```python
from build123d import *

# Parameters (mm, degrees)
F1_DEPTH = 50
F3_R     = 5
F4_DEPTH = 5
F5_DEPTH = 3


with BuildPart() as f1:
    # F0 (on Front) → F1 (new body)
    with BuildSketch(Plane.XZ):
        Polygon((86.1805300464, 183.2075325962), (81.2134853671, 183.7806531362), (60.0080253898, 0), (64.9750700692, -0.5731205399), align=None)
    extrude(amount=-F1_DEPTH)

    # F3 (on offset) → F4 (join)
    with BuildSketch(Plane.XZ.offset(-3)):
        with BuildLine():
            Line((45.1068913518, 1.7193616198), (60.0080253898, 0))
            Line((60.0080253898, 0), (63.4467486294, 29.8022680761))
            Line((63.4467486294, 29.8022680761), (48.5456145913, 31.5216296959))
            ThreePointArc((48.5456145913, 31.5216296959), (37.5053321271, 28.3729607019), (31.925118881, 18.3398568227))
            ThreePointArc((31.925118881, 18.3398568227), (35.0737879275, 7.2995748134), (45.1068913518, 1.7193616198))
        make_face()
        with Locations((46.8262529715, 16.6204956578)):
            Circle(F3_R, mode=Mode.SUBTRACT)
    extrude(amount=-F4_DEPTH)

    # F3 (on offset) → F5 (join)
    with BuildSketch(Plane.XZ.offset(-3)):
        with BuildLine():
            Line((45.1068913518, 1.7193616198), (60.0080253898, 0))
            Line((60.0080253898, 0), (63.4467486294, 29.8022680761))
            Line((63.4467486294, 29.8022680761), (48.5456145913, 31.5216296959))
            ThreePointArc((48.5456145913, 31.5216296959), (37.5053321271, 28.3729607019), (31.925118881, 18.3398568227))
            ThreePointArc((31.925118881, 18.3398568227), (35.0737879275, 7.2995748134), (45.1068913518, 1.7193616198))
        make_face()
        with Locations((46.8262529715, 16.6204956578)):
            Circle(F3_R, mode=Mode.SUBTRACT)
        with BuildLine():
            Line((48.5456145913, 31.5216296959), (63.4467486294, 29.8022680761))
            Line((63.4467486294, 29.8022680761), (81.2134853671, 183.7806531362))
            Line((81.2134853671, 183.7806531362), (51.411217291, 187.2193763757))
            Line((51.411217291, 187.2193763757), (31.925118881, 18.3398568227))
            ThreePointArc((31.925118881, 18.3398568227), (37.5053321271, 28.3729607019), (48.5456145913, 31.5216296959))
        make_face()
    extrude(amount=F5_DEPTH)


solid = f1.part
```
Geometry check sheet. Reference: the model listing, model coordinates, mm. Give positions to 0.01 mm unless a question says otherwise; leave off trailing zeros. Order: outer loops, then holes, each group sorted by start corner. A loop starts at its lowest first (then second) coordinate and runs counter-clockwise, first axis right, second up. Notation, with made-up numbers: (7.25, 75) - (18.25, 75) arc R23 ccw to (18.25, 93) - close; hole circle Ø2 at (67.5, 67.25). An arc over 180 degrees is marked (long way). Write item = value, one per line. Start each with the question number.
1) Scan lines: L1, parallel to Y at x = 57.5, z = 131.5; L2, parallel to X at y = 28.5, z = 149; L3, parallel to X at y = 47.5, z = 126. Record each from-to range of solid material in increasing order.
2) Section check A-A (x = 36.5). Enter the section's corners in (y, z), then the cut area to 3 significant figures.
3) Gauge pin test, flat ends, axial feed: pin 1 Ø5 at (x, z) = (51.5, 150) entering from +Y; pin 2 Ø16 at (x, z) = (45, 14.5) entering from +Y; pin 3 Ø1.5 at (y, z) = (20, 65) entering from +X; pin 4 Ø10 at (x, z) = (42, 73.5) entering from -Y. Record the tip position at first contact, or that the pin passes through.
4) Section check B-B (z = 135). Enter the section's corners in (x, y).
5) Section check C-C (y = 26). Enter the section's corners in (x, z), then the cut area to 3 significant figures.
6) Draft check along X on faces 1 (the flat face through (75.43, 24.65, 90.03)), 2 (the flat face through (56.1, 5.46, 30.65)), 3 (the flat face through (72, 50, 92)). Enter one of: released by +X, released by -X, zero draft, split by the parting line, or undercut.
Geometry check:
q1.L1 = 0 to 3
q1.L2 = 77.2 to 82.23
q1.L3 = 74.55 to 79.58
q2.outline = (0, 5.74) - (8, 5.74) - (8, 27.5) - (3, 27.5) - (3, 57.99) - (0, 57.99) - close
q2.area = 266 mm2
q3.pin_1 = 3
q3.pin_2 = 8
q3.pin_3 = 72.63
q3.pin_4 = 0
q4.outline = (45.39, 0) - (80.62, 0) - (80.62, 50) - (75.58, 50) - (75.58, 3) - (45.39, 3) - close
q5.outline = (60.01, 0) - (64.98, -0.57) - (86.18, 183.21) - (81.21, 183.78) - close
q5.area = 925 mm2
q6.face_1 = released by +X
q6.face_2 = undercut
q6.face_3 = zero draft
